Geometry check sheet. Reference: drawing and pictorial views, mm from the part's lowest x, y, z. A direction names the side the tool comes from. Give positions to 0.01 mm unless a question says otherwise; leave off trailing zeros. Order: outer loops, then holes, each group sorted by start corner. A loop starts at its lowest first (then second) coordinate and runs counter-clockwise, first axis right, second up. Notation, with made-up numbers: M 83,-11 L 109,-11 A17 ccw 109,9 Z; hole C -14.5,-6.5 d5. An arc over 180 degrees is marked long. Answer as CSV lines item,"result".
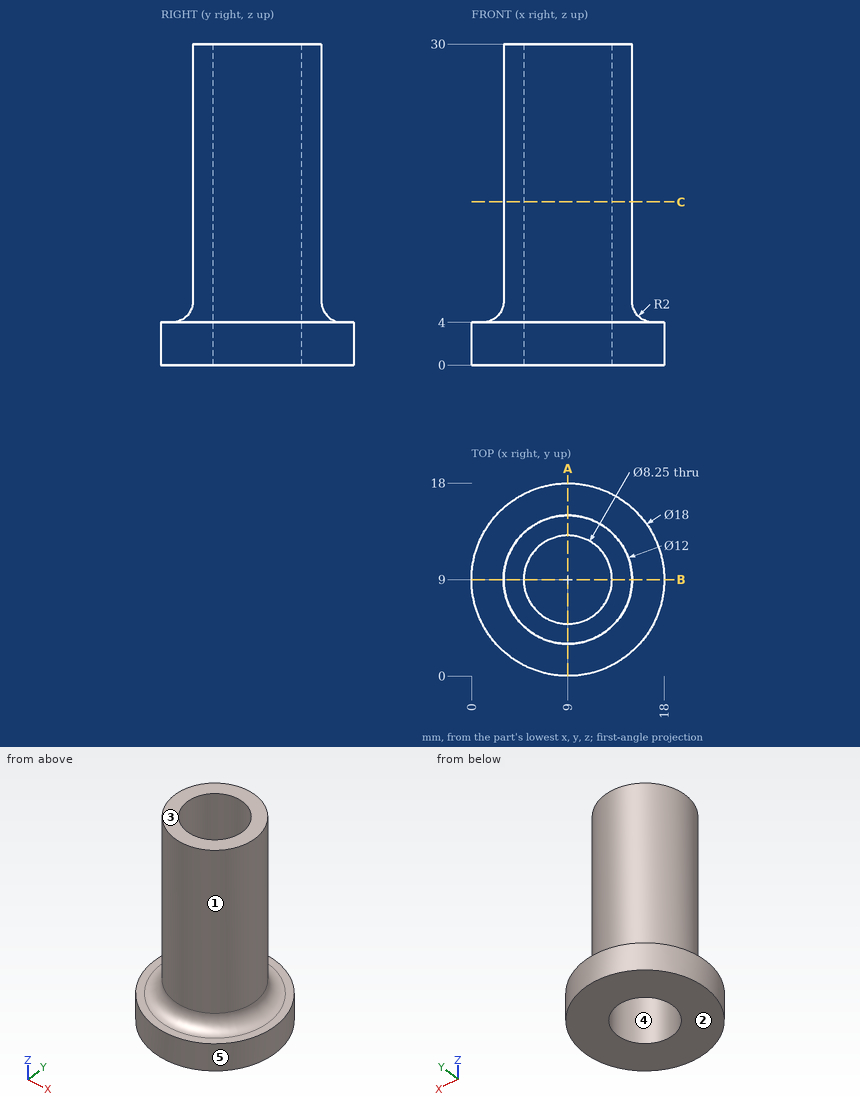
(1) Draft check along Y on the marked faces 3, 4 and 5. Enter one of: +Y half, -Y half, draft (parallel to the pull), parting line (faces both ways), or undercut.
The answers:
face 3,"draft"
face 4,"undercut"
face 5,"parting line"
(2) Section check A-A on x = 9. Enter the section's corners in (y, z) (3 decimals), then the cut area to 3 significant figures.
The answers:
outline,"M 0,0 L 4.875,0 L 4.875,30 L 3,30 L 3,6 A2 cw 1,4 L 0,4 Z; M 13.125,0 L 18,0 L 18,4 L 17,4 A2 cw 15,6 L 15,30 L 13.125,30 Z"
area,"138 mm2"
(3) Section check C-C on z = 15.25. Enter the section's corners in (x, y) (3 decimals).
The answers:
outline,"C 9,9 d12; hole C 9,9 d8.25"
(4) Material ranges on line 1 (Y direction, x = 9.25, z = 3); line 2 (Y direction, x = 9, z = 7.75) (3 decimals); line 3 (Z direction, x = 16.75, y = 5), recorded low to high.
The answers:
line 1,"y = 0 to 4.88, 13.12 to 18"
line 2,"y = 3 to 4.875, 13.125 to 15"
line 3,"z = 0 to 4"
(5) Tool access check on the marked faces 1 and 2. Record the directions out of +Z, -Z, +X, -X, +Y, -Y that give a thin tool (end or side, any length) a straight path to the whole face; none if there is none.
The answers:
face 1,"+Z"
face 2,"-Z, +X, -X, +Y, -Y"
(6) Gauge pin test, flat ends, axial feed: P1, Ø8, axis at x = 12, y = 12.5, coming from the -Z side; P2, Ø1, axis at y = 12.5, z = 7.5, coming from the -X side; P3, Ø1, axis at x = 10.5, z = 13.5, coming from the +Y side; P4, Ø3, axis at x = 14.5, z = 27, coming from the -Y side. Record the tip position at first contact, or that the pin passes through.
The answers:
P1,"stops at z = 0"
P2,"stops at x = 3.8"
P3,"stops at y = 14.92"
P4,"stops at y = 4.53"
